```python
from build123d import *

# Parameters (mm, degrees)
F0_W        = 36.83
F0_H        = 3.048
F1_DEPTH    = 10.414
F3_R        = 1.778
F4_T1_DEPTH = 45.9749047052
F5_DEPTH    = 25.4


# Not quite as in the source:
# - a fillet or chamfer that OpenCascade refuses, or shapes differently, is made with other operations: its cross-section is extruded or revolved along the edge and cut away or added


with BuildPart() as f1:
    # F0 (on Top) → F1 (new body)
    with BuildSketch(Plane.XY):
        with Locations((-0.254, 1.524)):
            Rectangle(F0_W, F0_H)
    extrude(amount=F1_DEPTH)

    # F3
    f3_edges = [f1.edges().sort_by_distance(p)[0] for p in [
        (-0.254, 3.048, 10.414),
    ]]
    fillet(f3_edges, radius=F3_R)

    # F4: chamfer of 1.778 on 1 edges, made by hand

    # F4_s2 → F4_t1 (cut)
    with BuildSketch(Plane.YZ.offset(-23.2414523526)):
        Polygon((1.778, 10.414), (0, 8.636), (0, 10.414), align=None)
    extrude(amount=F4_T1_DEPTH, mode=Mode.SUBTRACT)

    # F2 (on face) → F5 (cut)
    with BuildSketch(Plane.XZ):
        Polygon((-15.494, 8.8492954744), (-14.5906174209, 10.414), (-16.3973825791, 10.414), align=None)
        Polygon((-4.5039409051, 10.414), (-6.1640590949, 10.414), (-5.334, 8.9762954744), align=None)
        Polygon((5.8027060633, 10.414), (3.8492939367, 10.414), (4.826, 8.7222954744), align=None)
        Polygon((15.8160590949, 10.414), (14.1559409051, 10.414), (14.986, 8.9762954744), align=None)
    extrude(amount=-F5_DEPTH, mode=Mode.SUBTRACT)


solid = f1.part
```
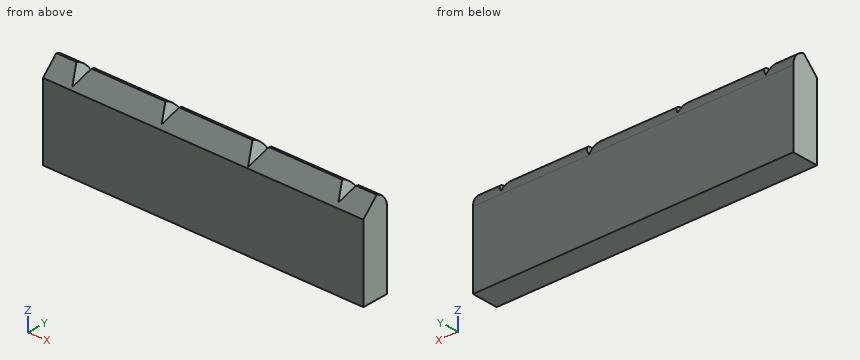
Source: CAD feature listing. Evaluate the final solid. Frame: model axes, mm. Give positions to 0.01 mm unless a question says otherwise; leave off trailing zeros. Order: outer loops, then holes, each group sorted by start corner. A loop starts at its lowest first (then second) coordinate and runs counter-clockwise, first axis right, second up.
(1) Material intervals for line 1 along Z through (x, y) = (-8, 2.6); line 2 along Z through (x, y) = (-14.5, 2.2); line 3 along Y through (x, z) = (1, 9.5), sorted ascending.
(2) Section query A-A (y = 1). Return the cut outline in (x, z).
(3) Section query C-C (y = 2.7). Return the cut outline in (x, z), plus the area to 3 significant figures.
(4) Section query B-B (x = -7). Return the cut outline in (y, z).
Outcome:
1. line 1: z = 0 to 9.82
1. line 2: z = 0 to 10.15
1. line 3: y = 0.86 to 2.82
2. outline: (-18.67, 0) - (18.16, 0) - (18.16, 9.64) - (15.37, 9.64) - (14.99, 8.98) - (14.61, 9.64) - (5.35, 9.64) - (4.83, 8.72) - (4.3, 9.64) - (-4.95, 9.64) - (-5.33, 8.98) - (-5.71, 9.64) - (-15.04, 9.64) - (-15.49, 8.85) - (-15.95, 9.64) - (-18.67, 9.64) - close
3. outline: (-18.67, 0) - (18.16, 0) - (18.16, 9.69) - (15.4, 9.69) - (14.99, 8.98) - (14.57, 9.69) - (5.39, 9.69) - (4.83, 8.72) - (4.27, 9.69) - (-4.92, 9.69) - (-5.33, 8.98) - (-5.75, 9.69) - (-15.01, 9.69) - (-15.49, 8.85) - (-15.98, 9.69) - (-18.67, 9.69) - close
3. area: 355 mm2
4. outline: (0, 0) - (3.05, 0) - (3.05, 8.64) arc R1.78 ccw to (1.72, 10.36) - (0, 8.64) - close
